```python
from build123d import *

# Parameters (mm, degrees)
SKETCH1_R                = 17.145
SKETCH1_R_2              = 2.5
BOSS_EXTRUDE1_DEPTH      = 3.81
BOSS_EXTRUDE2_DEPTH      = 45
BOSS_EXTRUDE2_DEPTH_BACK = 3.81
SKETCH2_R                = 7.62
SKETCH2_R_2              = 2.5
CUT_EXTRUDE2_DEPTH       = 118.102684
SKETCH6_R                = 8.89
SKETCH6_R_2              = 4.445
BOSS_EXTRUDE3_DEPTH      = 4.572
FILLET2_R                = 3.048


with BuildPart() as part:
    # Sketch1 → Boss-Extrude1 (new body)
    with BuildSketch(Plane(origin=(0, 0, 0), x_dir=(1, 0, 0), z_dir=(0, 1, 0))):
        with Locations(Location((0, 0, 0), (0, 0, 90))):
            Circle(SKETCH1_R)
        with Locations(Location((0, 9.5, 0), (0, 0, 90))):
            Circle(SKETCH1_R_2, mode=Mode.SUBTRACT)
        with Locations(Location((9.5, 0, 0), (0, 0, 90))):
            Circle(SKETCH1_R_2, mode=Mode.SUBTRACT)
        with Locations(Location((0, -9.5, 0), (0, 0, 90))):
            Circle(SKETCH1_R_2, mode=Mode.SUBTRACT)
        with Locations(Location((-9.5, 0, 0), (0, 0, 90))):
            Circle(SKETCH1_R_2, mode=Mode.SUBTRACT)
    extrude(amount=BOSS_EXTRUDE1_DEPTH)

    # Sketch2 → Boss-Extrude2 (add, two sides: drawn at the far end of the back side and taken through both)
    with BuildSketch(Plane(origin=(0, 3.81, 0), x_dir=(1, 0, 0), z_dir=(0, 1, 0)).offset(-BOSS_EXTRUDE2_DEPTH_BACK)):
        with BuildLine():
            Line((-96.52, -14.605), (96.52, -14.605))
            ThreePointArc((96.52, -14.605), (100.112102448, -13.117102448), (101.6, -9.525))
            Line((101.6, -9.525), (101.6, 9.525))
            ThreePointArc((101.6, 9.525), (100.112102448, 13.117102448), (96.52, 14.605))
            Line((96.52, 14.605), (-96.52, 14.605))
            ThreePointArc((-96.52, 14.605), (-100.112102448, 13.117102448), (-101.6, 9.525))
            Line((-101.6, 9.525), (-101.6, -9.525))
            ThreePointArc((-101.6, -9.525), (-100.112102448, -13.117102448), (-96.52, -14.605))
        make_face()
        with Locations(Location((-88.9, 0, 0), (0, 0, 270))):
            Circle(SKETCH2_R, mode=Mode.SUBTRACT)
        with Locations(Location((88.9, 0, 0), (0, 0, 270))):
            Circle(SKETCH2_R, mode=Mode.SUBTRACT)
        with Locations(Location((9.5, 0, 0), (0, 0, 90))):
            Circle(SKETCH2_R_2, mode=Mode.SUBTRACT)
        with Locations(Location((0, 9.5, 0), (0, 0, 90))):
            Circle(SKETCH2_R_2, mode=Mode.SUBTRACT)
        with Locations(Location((-9.5, 0, 0), (0, 0, 90))):
            Circle(SKETCH2_R_2, mode=Mode.SUBTRACT)
        with Locations(Location((0, -9.5, 0), (0, 0, 90))):
            Circle(SKETCH2_R_2, mode=Mode.SUBTRACT)
    extrude(amount=BOSS_EXTRUDE2_DEPTH + BOSS_EXTRUDE2_DEPTH_BACK)

    # Sketch5 → Cut-Extrude2 (cut, through all)
    with BuildSketch(Plane(origin=(0, 0, -14.605), x_dir=(-1, 0, 0), z_dir=(0, 0, -1))):
        Polygon((-76.2, 3.81), (0, 3.81), (76.2, 3.81), (76.2, 48.81), (-76.2, 48.81), align=None)
    extrude(amount=-CUT_EXTRUDE2_DEPTH, mode=Mode.SUBTRACT)

    # Sketch6 → Boss-Extrude3 (add)
    # profile 1 of 2: a face of its own
    with BuildSketch(Plane.XZ):
        with Locations((-88.9, 0)):
            Circle(SKETCH6_R)
        with Locations(Location((-88.9, 0, 0), (0, 0, 270))):
            Circle(SKETCH6_R_2, mode=Mode.SUBTRACT)
    # profile 2 of 2: a face of its own
    with BuildSketch(Plane.XZ):
        with Locations((88.9, 0)):
            Circle(SKETCH6_R)
        with Locations(Location((88.9, 0, 0), (0, 0, 270))):
            Circle(SKETCH6_R_2, mode=Mode.SUBTRACT)
    extrude(amount=-BOSS_EXTRUDE3_DEPTH)

    # Fillet2
    fillet2_edges = [part.edges().sort_by_distance(p)[0] for p in [
        (-76.2, 3.81, 0),
        (76.2, 3.81, 0),
    ]]
    fillet(fillet2_edges, radius=FILLET2_R)


solid = part.part
```
The listing builds one solid part. Answer for the finished solid, in the listing's coordinates (mm). A direction names the side the tool comes from. Round coordinates to 2 decimals unless told otherwise and drop trailing zeros. Order: outer loops, then holes, each group sorted by start corner. A loop starts at its lowest first (then second) coordinate and runs counter-clockwise, first axis right, second up. Notation, with made-up numbers: (88.5, 63.25) - (100.5, 63.25) arc R33 cw to (100.5, 94.25) - close; hole circle Ø11 at (57, 85). An arc over 180 degrees is marked (long way). Put each result on its own line as item: value. Start each with the question number.
(1) Find section D-D (x = 29.5). Give the vertices of the cut face in (y, z) (3 decimals), plus the area to 3 significant figures.
(2) Find section B-B (y = 26). Give the vertices of the cut face in (x, z) (3 decimals).
(3) Determine the mould class of faces 6 (the flat face through (101.6, 24, 0)), 7 (the cylindrical face through (0.132, 1.878, -17.144)), 8 (the flat face through (76.2, 28, 0)) for opening direction X: released by +X, released by -X, zero draft, split by the parting line, or undercut.
(4) For faces 1 (the cylindrical face through (-96.34, 26.38, -1.65)), 2 (the flat face through (1, 3.81, 0)), 3 (the flat face through (-79, 19, 14.605)), 4 (the flat face through (79, 19, -14.605)), 5 (the flat face through (78, 19, 14.605)), determine the directions among +Z, -Z, +X, -X, +Y, -Y from which every point of the face is accessible in a straight line to the end or side of a thin tool.
(5) Find section A-A (z = 0). State how many separate pieces and enclosed holes the cut face has, plus the area to 3 significant figures.
(6) Straight lines are drawn through the part: probe 1 along X at (y, z) = (16.5, -0.5); probe 2 along X at (y, z) = (1.7, 0) (3 decimals); probe 3 along X at (y, z) = (35.5, 9.5). For each, find the intervals that lie inside material, in ascending order. Write a range as from..to.
(7) Given P1, Ø11.5, axis at x = 88.9, z = 0, coming from the +Y side; P2, Ø1.5, axis at x = -58.5, z = -9.5, coming from the +Y side; P3, Ø6, axis at x = -10.5, y = 5.5, coming from the -Z side, each flat-ended and moving along its own axis, determine where each tip first touches the part or whether it passes through.
(8) Find section C-C (x = -88.9). Give the vertices of the cut face in (y, z) (3 decimals).
Reply:
1. outline: (0, -14.605) - (3.81, -14.605) - (3.81, 14.605) - (0, 14.605) - close
1. area: 111 mm^2
2. outline: (-101.6, -9.525) arc R5.08 ccw to (-96.52, -14.605) - (-76.2, -14.605) - (-76.2, 14.605) - (-96.52, 14.605) arc R5.08 ccw to (-101.6, 9.525) - close; (76.2, -14.605) - (96.52, -14.605) arc R5.08 ccw to (101.6, -9.525) - (101.6, 9.525) arc R5.08 ccw to (96.52, 14.605) - (76.2, 14.605) - close; hole circle Ø15.24 at (-88.9, 0); hole circle Ø15.24 at (88.9, 0)
3. face 6: released by +X
3. face 7: split by the parting line
3. face 8: undercut
4. face 1: +Y
4. face 2: +Z, -Z, +Y
4. face 3: +Z, -X, +Y, -Y
4. face 4: -Z, +X, +Y, -Y
4. face 5: +Z, +X, +Y, -Y
5. separate pieces: 5
5. enclosed holes: 0
5. area: 1,600 mm^2
6. probe 1: -101.6..-96.5, -81.3..-76.2, 76.2..81.3, 96.5..101.6
6. probe 2: -101.6..-93.345, -84.455..-12, -7..7, 12..84.455, 93.345..101.6
6. probe 3: -101.6..-76.2, 76.2..101.6
7. P1: y = 4.57
7. P2: y = 3.81
7. P3: z = -15.15
8. outline: (0, -14.605) - (48.81, -14.605) - (48.81, -7.62) - (4.572, -7.62) - (4.572, -4.445) - (0, -4.445) - close; (0, 4.445) - (4.572, 4.445) - (4.572, 7.62) - (48.81, 7.62) - (48.81, 14.605) - (0, 14.605) - close
